Part model, mm, in its own coordinate system. Face numbers are marked on the shaded views. A direction names the side the tool comes from. Give positions to 0.01 mm unless a question says otherwise; leave off trailing zeros. Order: outer loops, then holes, each group sorted by start corner. A loop starts at its lowest first (then second) coordinate and runs counter-clockwise, first axis right, second up. Notation, with made-up numbers: (-23, 75) -> (27, 75) arc R17 ccw to (27, 108) -> close; hole circle Ø6 at (70, 0). An arc over 180 degrees is marked (long way). Write item = value, one per line. Start each with the question number.
(1) Which spindle directions (+Z, -Z, +X, -X, +Y, -Y) get a long thin tool onto all of the face, cutting with end or side? Do the marked faces 3 and 4. Say none if no direction does.
(2) Saw through at A-A, the plane y = 17. List the corners of the cut face in (x, z).
(3) Two-plate mould, pull along X, no slides. Class the marked faces 1 and 2: pulls with the +X half, pulls with the -X half, needs draft (parallel to the pull), parting line crosses it, or undercut.
(4) Saw through at B-B, the plane x = 6. List the corners of the cut face in (y, z), then the cut area to 3 significant figures.
(5) Probe line 1 along Z through (x, y) = (57.5, -5); line 2 along X through (y, z) = (167.5, 180.5); line 3 along X through (y, z) = (-180, 124). List the from-to ranges inside material, lowest first. Write a range as from..to.
(6) Saw through at C-C, the plane z = 236.5. List the corners of the cut face in (x, y), then the cut area to 3 significant figures.
(7) Flat gauge pins, fed straight in: pin 1 (3 mm diameter, centred on y = 122, z = 199, fed in from +X); pin 2 (3 mm diameter, centred on x = 28, y = 89.5, fed in from -Z); pin 3 (22 mm diameter, centred on x = 25.5, z = 208, fed in from -Y). Where does each tip first touch, or does it go through?
from build123d import *

# Parameters (mm, degrees)
F1_W     = 400
F1_H     = 400
F2_DEPTH = 25
F4_DEPTH = 375
F6_W     = 350
F6_H     = 350
F7_DEPTH = 20


with BuildPart() as f2:
    # F1 (on offset) → F2 (new body)
    with BuildSketch(Plane.XY.offset(400)):
        Rectangle(F1_W, F1_H)
    extrude(amount=-F2_DEPTH)

    # F3 (on face) → F4 (join)
    with BuildSketch(Plane(origin=(0, 0, 375), x_dir=(1, 0, 0), z_dir=(0, 0, -1))):
        Polygon((-200, 200), (-200, 150), (-175, 150), (-175, 175), (-150, 175), (-150, 200), align=None)
        Polygon((175, 150), (200, 150), (200, 200), (150, 200), (150, 175), (175, 175), align=None)
        Polygon((-150, -175), (-175, -175), (-175, -150), (-200, -150), (-200, -200), (-150, -200), align=None)
        Polygon((200, -200), (200, -150), (175, -150), (175, -175), (150, -175), (150, -200), align=None)
    extrude(amount=F4_DEPTH)

    # F6 (on offset) → F7 (join)
    with BuildSketch(Plane.XY.offset(200)):
        with Locations((0.264752, 0.58246)):
            Rectangle(F6_W, F6_H)
    extrude(amount=F7_DEPTH)


solid = f2.part
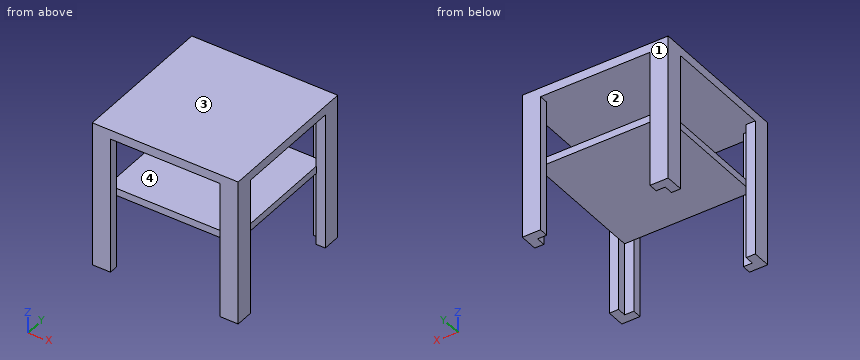
Results list:
q1.face_3 = +Z, +X, -X, +Y, -Y
q1.face_4 = none
q2.outline = (-200, 375) -> (200, 375) -> (200, 400) -> (-200, 400) -> close; (-174.74, 200) -> (175.26, 200) -> (175.26, 220) -> (-174.74, 220) -> close
q3.face_1 = needs draft
q3.face_2 = undercut
q4.outline = (-200, 375) -> (200, 375) -> (200, 400) -> (-200, 400) -> close; (-174.42, 200) -> (175.58, 200) -> (175.58, 220) -> (-174.42, 220) -> close
q4.area = 17,000 mm^2
q5.line_1 = 200..220, 375..400
q5.line_2 = -200..-175, 175..200
q5.line_3 = -200..-150, 150..200
q6.outline = (-200, -200) -> (-150, -200) -> (-150, -175) -> (-175, -175) -> (-175, -150) -> (-200, -150) -> close; (-200, 150) -> (-175, 150) -> (-175, 175) -> (-150, 175) -> (-150, 200) -> (-200, 200) -> close; (150, -200) -> (200, -200) -> (200, -150) -> (175, -150) -> (175, -175) -> (150, -175) -> close; (150, 175) -> (175, 175) -> (175, 150) -> (200, 150) -> (200, 200) -> (150, 200) -> close
q6.area = 7,500 mm^2
q7.pin_1 = 175.26
q7.pin_2 = 200
q7.pin_3 = -174.42
